```python
from build123d import *

# Parameters (mm, degrees)
SKETCH1_R                      = 15.35
BOSS_EXTRUDE1_DEPTH            = 2.71
SKETCH2_R                      = 2.685
BOSS_EXTRUDE2_DEPTH            = 1.2
DOME1_FACE_RADIUS              = 2.685
DOME1_HEIGHT                   = 0.6
CIRPATTERN1_COUNT              = 3
CIRPATTERN1_COPY_1_FACE_RADIUS = 2.685
CIRPATTERN1_COPY_1_HEIGHT      = 0.6
CIRPATTERN1_COPY_2_FACE_RADIUS = 2.685
CIRPATTERN1_COPY_2_HEIGHT      = 0.6
BOSS_EXTRUDE3_START            = 2.55
SKETCH3_W                      = 5.5
SKETCH3_H                      = 4.2
SKETCH3_W_2                    = 1.5
SKETCH3_H_2                    = 2.8
BOSS_EXTRUDE3_DEPTH            = 2.55
SKETCH4_W                      = 5.5
SKETCH4_H                      = 4.2
BOSS_EXTRUDE4_DEPTH            = 1.44
CHIP_DEPTH                     = 1.7018
BOSS_EXTRUDE5_DEPTH            = 2.032
BOSS_EXTRUDE6_START            = 6.37794
SKETCH7_R                      = 16.5862
SKETCH7_R_2                    = 15.35
BOSS_EXTRUDE6_DEPTH            = 6.37794
BOSS_EXTRUDE7_START            = -8.40994
SKETCH8_R                      = 1.397
BOSS_EXTRUDE7_DEPTH            = 8.40994
SKETCH9_R                      = 2.5443
CUT_EXTRUDE1_DEPTH             = 5.86994
CUT_EXTRUDE4_REACH             = 31.486
FILLET1_R                      = 1.27


with BuildPart() as part:
    # Sketch1 → Boss-Extrude1 (new body)
    with BuildSketch(Plane(origin=(0, 0, 0), x_dir=(1, 0, 0), z_dir=(0, 1, 0))):
        with Locations(Location((0, 0, 0), (0, 0, 270))):
            Circle(SKETCH1_R)
    extrude(amount=BOSS_EXTRUDE1_DEPTH)

    # Sketch2 → Boss-Extrude2 (add)
    with BuildSketch(Plane(origin=(0, 2.71, 0), x_dir=(-1, 0, 0), z_dir=(0, 1, 0))):
        with Locations(Location((-5.5, 9.526279442, 0), (0, 0, 90))):
            Circle(SKETCH2_R)
    boss_extrude2 = extrude(amount=BOSS_EXTRUDE2_DEPTH)

    # Dome1: a dome of height H over a round flat face of radius A is a cap of a sphere of radius (A * A + H * H) / (2 * H)
    dome1_r = (DOME1_FACE_RADIUS * DOME1_FACE_RADIUS + DOME1_HEIGHT * DOME1_HEIGHT) / (2 * DOME1_HEIGHT)
    dome1_base = Plane((5.5, 3.91, 9.526279442), z_dir=(0, 1, 0))
    with Locations(dome1_base.offset(DOME1_HEIGHT - dome1_r)):
        dome1_ball = Sphere(dome1_r, mode=Mode.PRIVATE)
    add(split(dome1_ball, bisect_by=dome1_base, keep=Keep.TOP, mode=Mode.PRIVATE))

    # CirPattern1: Boss-Extrude2 ×3 about axis
    cirpattern1_axis = Axis((0, 0, 0), (0, 1, 0))
    for i in range(1, CIRPATTERN1_COUNT):
        add(boss_extrude2.rotate(cirpattern1_axis, i * 360 / CIRPATTERN1_COUNT))

    # CirPattern1 copy 1: a dome of height H over a round flat face of radius A is a cap of a sphere of radius (A * A + H * H) / (2 * H)
    cirpattern1_copy_1_r = (CIRPATTERN1_COPY_1_FACE_RADIUS * CIRPATTERN1_COPY_1_FACE_RADIUS + CIRPATTERN1_COPY_1_HEIGHT * CIRPATTERN1_COPY_1_HEIGHT) / (2 * CIRPATTERN1_COPY_1_HEIGHT)
    cirpattern1_copy_1_base = Plane((5.5, 3.91, -9.526279442), z_dir=(0, 1, 0))
    with Locations(cirpattern1_copy_1_base.offset(CIRPATTERN1_COPY_1_HEIGHT - cirpattern1_copy_1_r)):
        cirpattern1_copy_1_ball = Sphere(cirpattern1_copy_1_r, mode=Mode.PRIVATE)
    add(split(cirpattern1_copy_1_ball, bisect_by=cirpattern1_copy_1_base, keep=Keep.TOP, mode=Mode.PRIVATE))

    # CirPattern1 copy 2: a dome of height H over a round flat face of radius A is a cap of a sphere of radius (A * A + H * H) / (2 * H)
    cirpattern1_copy_2_r = (CIRPATTERN1_COPY_2_FACE_RADIUS * CIRPATTERN1_COPY_2_FACE_RADIUS + CIRPATTERN1_COPY_2_HEIGHT * CIRPATTERN1_COPY_2_HEIGHT) / (2 * CIRPATTERN1_COPY_2_HEIGHT)
    cirpattern1_copy_2_base = Plane((-11, 3.91, 0), z_dir=(0, 1, 0))
    with Locations(cirpattern1_copy_2_base.offset(CIRPATTERN1_COPY_2_HEIGHT - cirpattern1_copy_2_r)):
        cirpattern1_copy_2_ball = Sphere(cirpattern1_copy_2_r, mode=Mode.PRIVATE)
    add(split(cirpattern1_copy_2_ball, bisect_by=cirpattern1_copy_2_base, keep=Keep.TOP, mode=Mode.PRIVATE))

    # Sketch3 → Boss-Extrude3 (add)
    with BuildSketch(Plane.XZ.offset(BOSS_EXTRUDE3_START)):
        with Locations((0, 13.05)):
            Rectangle(SKETCH3_W, SKETCH3_H)
        with Locations((0, -13.05)):
            Rectangle(SKETCH3_W, SKETCH3_H)
        with Locations((3.5, 13.05)):
            Rectangle(SKETCH3_W_2, SKETCH3_H_2)
        with Locations((-3.5, 13.05)):
            Rectangle(SKETCH3_W_2, SKETCH3_H_2)
        with Locations((3.5, -13.05)):
            Rectangle(SKETCH3_W_2, SKETCH3_H_2)
        with Locations((-3.5, -13.05)):
            Rectangle(SKETCH3_W_2, SKETCH3_H_2)
        with BuildLine():
            Line((2.75, 15.101655538), (2.75, 15.15))
            Line((2.75, 15.15), (2.469817807, 15.15))
            ThreePointArc((2.469817807, 15.15), (2.610020839, 15.126476497), (2.75, 15.101655538))
        make_face()
        with BuildLine():
            ThreePointArc((-2.75, 15.101655538), (-2.610020839, 15.126476497), (-2.469817807, 15.15))
            Line((-2.469817807, 15.15), (-2.75, 15.15))
            Line((-2.75, 15.15), (-2.75, 15.101655538))
        make_face()
        with BuildLine():
            ThreePointArc((-2.469817807, -15.15), (-2.610020839, -15.126476497), (-2.75, -15.101655538))
            Line((-2.75, -15.101655538), (-2.75, -15.15))
            Line((-2.75, -15.15), (-2.469817807, -15.15))
        make_face()
        with BuildLine():
            Line((2.75, -15.15), (2.75, -15.101655538))
            ThreePointArc((2.75, -15.101655538), (2.610020839, -15.126476497), (2.469817807, -15.15))
            Line((2.469817807, -15.15), (2.75, -15.15))
        make_face()
    extrude(amount=-BOSS_EXTRUDE3_DEPTH)

    # Sketch4 → Boss-Extrude4 (add)
    with BuildSketch(Plane.XZ.offset(2.55)):
        Polygon((-2.75, 10.95), (2.75, 10.95), (2.75, 11.65), (2.75, 14.45), (2.75, 15.15), (-2.75, 15.15), (-2.75, 14.45), (-2.75, 11.65), align=None)
        with Locations((0, -13.05)):
            Rectangle(SKETCH4_W, SKETCH4_H)
    extrude(amount=BOSS_EXTRUDE4_DEPTH)

    # Sketch5 → Chip (add)
    with BuildSketch(Plane.XZ):
        Polygon((-5.1644, -9.425953844), (-2.016601499, -2.878979584), (-8.014179317, 0.004667994), (-11.161977818, -6.542306266), align=None)
    extrude(amount=CHIP_DEPTH)

    # Sketch6 → Boss-Extrude5 (add)
    with BuildSketch(Plane.XZ.offset(2.55)):
        with BuildLine():
            Line((-3.175, 16.279478046), (-3.175, 10.525))
            Line((-3.175, 10.525), (3.175, 10.525))
            Line((3.175, 10.525), (3.175, 16.279478046))
            ThreePointArc((3.175, 16.279478046), (16.5862, 0), (3.175, -16.279478046))
            Line((3.175, -16.279478046), (3.175, -10.525))
            Line((3.175, -10.525), (-3.175, -10.525))
            Line((-3.175, -10.525), (-3.175, -16.279478046))
            ThreePointArc((-3.175, -16.279478046), (-16.5862, 0), (-3.175, 16.279478046))
        make_face()
    extrude(amount=BOSS_EXTRUDE5_DEPTH)

    # Sketch7 → Boss-Extrude6 (add)
    with BuildSketch(Plane(origin=(0, -2.55, 0), x_dir=(1, 0, 0), z_dir=(0, 1, 0)).offset(BOSS_EXTRUDE6_START)):
        with Locations(Location((0, 0, 0), (0, 0, 270))):
            Circle(SKETCH7_R)
        with Locations(Location((0, 0, 0), (0, 0, 270))):
            Circle(SKETCH7_R_2, mode=Mode.SUBTRACT)
    extrude(amount=-BOSS_EXTRUDE6_DEPTH)

    # Sketch8 → Boss-Extrude7 (add)
    # profile 1 of 2: a face of its own
    with BuildSketch(Plane.XZ.offset(4.582).offset(BOSS_EXTRUDE7_START)):
        with BuildLine():
            ThreePointArc((-16.294154443, -3.0988), (-16.5862, 0), (-16.294154443, 3.0988))
            Line((-16.294154443, 3.0988), (-21.46935, 3.0988))
            Line((-21.46935, 3.0988), (-21.46935, -3.0988))
            Line((-21.46935, -3.0988), (-16.294154443, -3.0988))
        make_face()
        with Locations(Location((-18.3642, 0, 0), (0, 0, 270))):
            Circle(SKETCH8_R, mode=Mode.SUBTRACT)
    # profile 2 of 2: a face of its own
    with BuildSketch(Plane.XZ.offset(4.582).offset(BOSS_EXTRUDE7_START)):
        with BuildLine():
            Line((21.46935, 3.0988), (16.294154443, 3.0988))
            ThreePointArc((16.294154443, 3.0988), (16.5862, 0), (16.294154443, -3.0988))
            Line((16.294154443, -3.0988), (21.46935, -3.0988))
            Line((21.46935, -3.0988), (21.46935, 3.0988))
        make_face()
        with Locations(Location((18.3642, 0, 0), (0, 0, 270))):
            Circle(SKETCH8_R, mode=Mode.SUBTRACT)
    extrude(amount=BOSS_EXTRUDE7_DEPTH)

    # Sketch9 → Cut-Extrude1 (cut)
    with BuildSketch(Plane(origin=(0, 3.82794, 0), x_dir=(1, 0, 0), z_dir=(0, 1, 0))):
        with Locations(Location((-18.3642, 0, 0), (0, 0, 270))):
            Circle(SKETCH9_R)
    cut_extrude1 = extrude(amount=-CUT_EXTRUDE1_DEPTH, mode=Mode.SUBTRACT)

    # Cut-Extrude4: up to this face of the body (flat: up to its plane)
    cut_extrude4_end = Plane(part.part.faces().sort_by_distance((-18.881752221, -0.37703, -3.0988))[0])
    # Sketch10 → Cut-Extrude4 (cut, up to the picked face)
    with BuildSketch(Plane.XY.offset(3.0988), mode=Mode.PRIVATE) as cut_extrude4_sk1:
        Polygon((-21.46935, -2.042), (-18.39595, -2.042), (-16.294154443, 3.82794), (-21.46935, 3.82794), align=None)
    cut_extrude4_tool1 = split(extrude(cut_extrude4_sk1.sketch, amount=-CUT_EXTRUDE4_REACH, mode=Mode.PRIVATE), bisect_by=cut_extrude4_end, keep=Keep.BOTH, mode=Mode.PRIVATE)
    cut_extrude4 = cut_extrude4_tool1.solids().sort_by(Axis((-19.362572, 1.142253, 3.0988), (0, 0, -1)))[0]
    add(cut_extrude4, mode=Mode.SUBTRACT)

    # Mirror2: Cut-Extrude1, Cut-Extrude4 across plane
    add(cut_extrude1.mirror(Plane(origin=(0, 0, 0), x_dir=(0, 0, 1), z_dir=(1, 0, 0))), mode=Mode.SUBTRACT)
    add(cut_extrude4.mirror(Plane(origin=(0, 0, 0), x_dir=(0, 0, 1), z_dir=(1, 0, 0))), mode=Mode.SUBTRACT)

    # Fillet1
    fillet1_edges = [part.edges().sort_by_distance(p)[0] for p in [
        (16.294154443, -0.37703, -3.0988),
        (16.294154443, -0.37703, 3.0988),
        (-16.294154443, 0.63897, -3.0988),
        (-16.294154443, 0.63897, 3.0988),
        (-21.46935, -3.312, 3.0988),
        (-21.46935, -3.312, -3.0988),
        (21.46935, -3.312, 3.0988),
        (21.46935, -3.312, -3.0988),
    ]]
    fillet(fillet1_edges, radius=FILLET1_R)


solid = part.part
```
Read the model definition and answer for the solid it produces. Units are mm, in the model's axes. A direction names the side the tool comes from. Coordinates: 2 decimals unless noted, no trailing zeros. Write each loop counter-clockwise with the first axis right and the second up, starting at its lowest first coordinate (ties: lowest second). Pieces come first, ordered by that corner, then holes. Notation, with made-up numbers: (49.5, -35) -> (101.5, -35) arc R22 ccw to (101.5, -24) -> close; hole circle Ø2 at (32.5, 20.25). An arc over 180 degrees is marked (long way). Answer as a JSON object with one key per item and string values.
Q1. A tool of negligible diameter and unlimited length cuts with its end or side. For faces 4 (the flat face through (-20, -2.042, 0)), 5 (the flat face through (-3.613, -0.839, -6.198)), 6 (the flat face through (-3.175, -4, -13)), 7 (the cylindrical face through (-13.4, 3.3, 1.2)), from which of +Z, -Z, +X, -X, +Y, -Y can it reach the whole face along a straight path? Write none if from no direction.
The answers:
{"face 4": "-X, +Y", "face 5": "none", "face 6": "-Z, -Y", "face 7": "+Y"}
Q2. The part is cut by section B-B on z = 10. Give the vertices of the cut face in (x, y).
The answers:
{"outline": "(-13.23, -4.58) -> (13.23, -4.58) -> (13.23, 3.83) -> (11.65, 3.83) -> (11.65, 2.71) -> (8.14, 2.71) -> (8.14, 3.91) arc R6.29 ccw to (2.86, 3.91) -> (2.86, 2.71) -> (-11.65, 2.71) -> (-11.65, 3.83) -> (-13.23, 3.83) -> close; hole (-11.65, -2.55) -> (11.65, -2.55) -> (11.65, 0) -> (-11.65, 0) -> close"}
Q3. Consider line 1 (X direction, y = -3.25, z = 0); line 2 (Y direction, x = 11.5, z = -6); line 3 (X direction, y = -2, z = 11). Determine where each line is inside the solid, lowest interval first. Write a range as [from, to].
The answers:
{"line 1": "x = [-21.47, -19.76], [-16.97, 16.97], [19.76, 21.47]", "line 2": "y = [-4.58, -2.55], [0, 2.71]", "line 3": "x = [-12.41, -10.71], [-2.75, 2.75], [10.71, 12.41]"}
Q4. Determine the mould class of faces 1 (the flat face through (-18, -3, -3.099)), 2 (the flat face through (3.175, -4, -13)), 3 (the flat face through (-21.469, -3, 0)) for opening direction X: pulls with the +X half, pulls with the -X half, needs draft (parallel to the pull), parting line crosses it, or undercut.
The answers:
{"face 1": "needs draft", "face 2": "undercut", "face 3": "pulls with the -X half"}
Q5. The part is cut by section C-C on x = 5.5. Give the vertices of the cut face in (y, z).
The answers:
{"outline": "(-4.58, -15.65) -> (3.83, -15.65) -> (3.83, -14.33) -> (2.71, -14.33) -> (2.71, -12.21) -> (3.91, -12.21) arc R6.31 ccw to (3.91, -6.84) -> (2.71, -6.84) -> (2.71, 6.84) -> (3.91, 6.84) arc R6.31 ccw to (3.91, 12.21) -> (2.71, 12.21) -> (2.71, 14.33) -> (3.83, 14.33) -> (3.83, 15.65) -> (-4.58, 15.65) -> close; hole (-2.55, -14.33) -> (0, -14.33) -> (0, 14.33) -> (-2.55, 14.33) -> close"}
Q6. Flat-ended cylindrical pins translate along their axes: pin 1 Ø2 at (x, z) = (11.5, -1) entering from +Y; pin 2 Ø3 at (x, y) = (-18.5, -2.5) entering from +Z; pin 3 Ø1.2 at (y, z) = (-2.5, -13) entering from -X. Find the tip coordinate at first contact, or state that the pin passes through.
The answers:
{"pin 1": "stops at y = 2.71", "pin 2": "stops at z = 3.14", "pin 3": "stops at x = -11.02"}
Q7. The part is cut by section D-D on y = 1.5. Give the vertices of the cut face in (x, z).
The answers:
{"outline": "(-17.13, -3.11) arc R1.27 cw to (-16.08, -4.06) arc R16.59 ccw to (16.08, -4.06) arc R1.27 cw to (17.13, -3.11) -> (17.13, -2.22) arc R2.54 cw to (17.13, 2.22) -> (17.13, 3.11) arc R1.27 cw to (16.08, 4.06) arc R16.59 ccw to (-16.08, 4.06) arc R1.27 cw to (-17.13, 3.11) -> (-17.13, 2.22) arc R2.54 cw to (-17.13, -2.22) -> close"}
Q8. The part is cut by section A-A on x = 0. Give the vertices of the cut face in (y, z) (3 decimals).
The answers:
{"outline": "(-4.582, -10.525) -> (-2.55, -10.525) -> (-2.55, 10.525) -> (-4.582, 10.525) -> close; (-3.99, -15.15) -> (0, -15.15) -> (0, -15.35) -> (-2.55, -15.35) -> (-2.55, -16.586) -> (3.828, -16.586) -> (3.828, -15.35) -> (2.71, -15.35) -> (2.71, 15.35) -> (3.828, 15.35) -> (3.828, 16.586) -> (-2.55, 16.586) -> (-2.55, 15.35) -> (0, 15.35) -> (0, 15.15) -> (-3.99, 15.15) -> (-3.99, 10.95) -> (0, 10.95) -> (0, -10.95) -> (-3.99, -10.95) -> close"}
